The drawing under review shows one solid part. Ordinate dimensions are in mm from its lowest x, y, z. A direction names the side the tool comes from. Give positions to 0.01 mm unless a question says otherwise; leave off trailing zeros. Write each loop counter-clockwise with the first axis right and the second up, starting at its lowest first coordinate (ties: lowest second). Pieces come first, ordered by that corner, then holes. Notation, with made-up numbers: (5.25, 75.25) -> (59.25, 75.25) arc R21 ccw to (59.25, 86.25) -> close; hole circle Ø3 at (42, 62). An arc over 180 degrees is marked (long way). Answer as a JSON object with one key per item and string values.
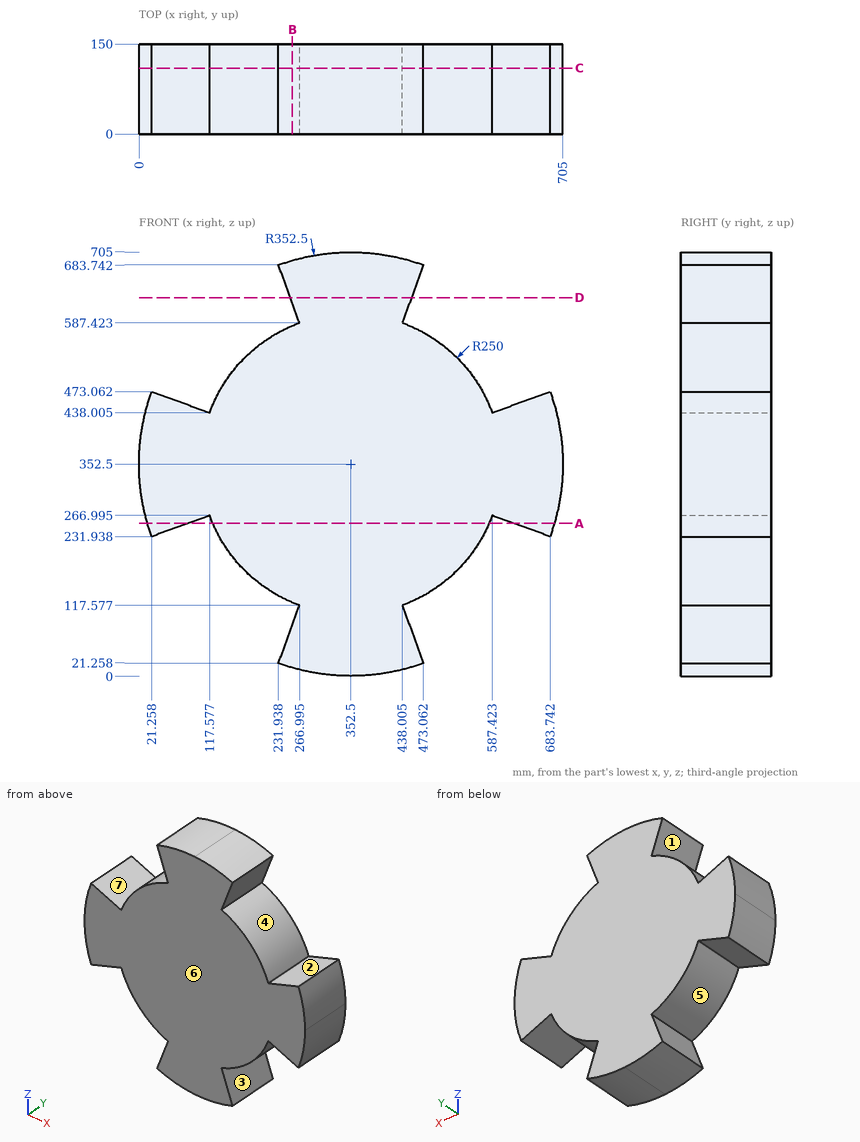
(1) For line 1 along Z through (x, y) = (40.5, 36); line 2 along X through (y, z) = (68, 553); line 3 along X through (y, z) = (91.5, 548), list the stretches that pass through material, from the lowest coordinate up.
Here are the results:
{"line 1": "z = 238.94 to 466.06", "line 2": "x = 203.17 to 501.83", "line 3": "x = 196.68 to 508.32"}
(2) For the marked faces 1, 2, 3 and 4, list the 3-axis set-ups (+Z, -Z, +X, -X, +Y, -Y) from which the entire face can be reached by the end or side of a thin tool; tool diameter is ignored.
Here are the results:
{"face 1": "-X, +Y, -Y", "face 2": "+Z, +Y, -Y", "face 3": "+X, +Y, -Y", "face 4": "+Y, -Y"}
(3) We need section B-B, the plane x = 255. State the section outline as (y, z) points, then the cut area to 3 significant figures.
Here are the results:
{"outline": "(0, 13.75) -> (150, 13.75) -> (150, 84.62) -> (0, 84.62) -> close; (0, 122.3) -> (150, 122.3) -> (150, 582.7) -> (0, 582.7) -> close; (0, 620.38) -> (150, 620.38) -> (150, 691.25) -> (0, 691.25) -> close", "area": "90,300 mm²"}
(4) We need section D-D, the plane z = 629.5. State the section outline as (x, y) points.
Here are the results:
{"outline": "(251.68, 0) -> (453.32, 0) -> (453.32, 150) -> (251.68, 150) -> close"}
(5) We need section A-A, the plane z = 254. State the section outline as (x, y) points.
Here are the results:
{"outline": "(14.04, 0) -> (81.87, 0) -> (81.87, 150) -> (14.04, 150) -> close; (122.72, 0) -> (582.28, 0) -> (582.28, 150) -> (122.72, 150) -> close; (623.13, 0) -> (690.96, 0) -> (690.96, 150) -> (623.13, 150) -> close"}
(6) We need section C-C, the plane y = 110. State the section outline as (x, z) points (1 decimal).
Here are the results:
{"outline": "(21.3, 231.9) -> (117.6, 267) arc R250 ccw to (267, 117.6) -> (231.9, 21.3) arc R352.5 ccw to (473.1, 21.3) -> (438, 117.6) arc R250 ccw to (587.4, 267) -> (683.7, 231.9) arc R352.5 ccw to (683.7, 473.1) -> (587.4, 438) arc R250 ccw to (438, 587.4) -> (473.1, 683.7) arc R352.5 ccw to (231.9, 683.7) -> (267, 587.4) arc R250 ccw to (117.6, 438) -> (21.3, 473.1) arc R352.5 ccw to start"}
(7) Clearance check with flat-ended pins moving along their axes: pin 1 (4 mm diameter, centred on y = 63, z = 502.5, fed in from -X) (1 decimal); pin 2 (1.5 mm diameter, centred on y = 41.5, z = 220.5, fed in from +X) (1 decimal); pin 3 (5 mm diameter, centred on x = 557.5, y = 29, fed in from -Z). State where each tip first meets the part, or that it passes through.
Here are the results:
{"pin 1": "stops at x = 151", "pin 2": "stops at x = 565.3", "pin 3": "stops at z = 205.89"}
(8) The part is to be moulded in two halves that separate along Z. For the marked faces 5, 6 and 7, say which applies: +Z half, -Z half, draft (parallel to the pull), parting line (faces both ways), or undercut.
Here are the results:
{"face 5": "undercut", "face 6": "draft", "face 7": "+Z half"}
